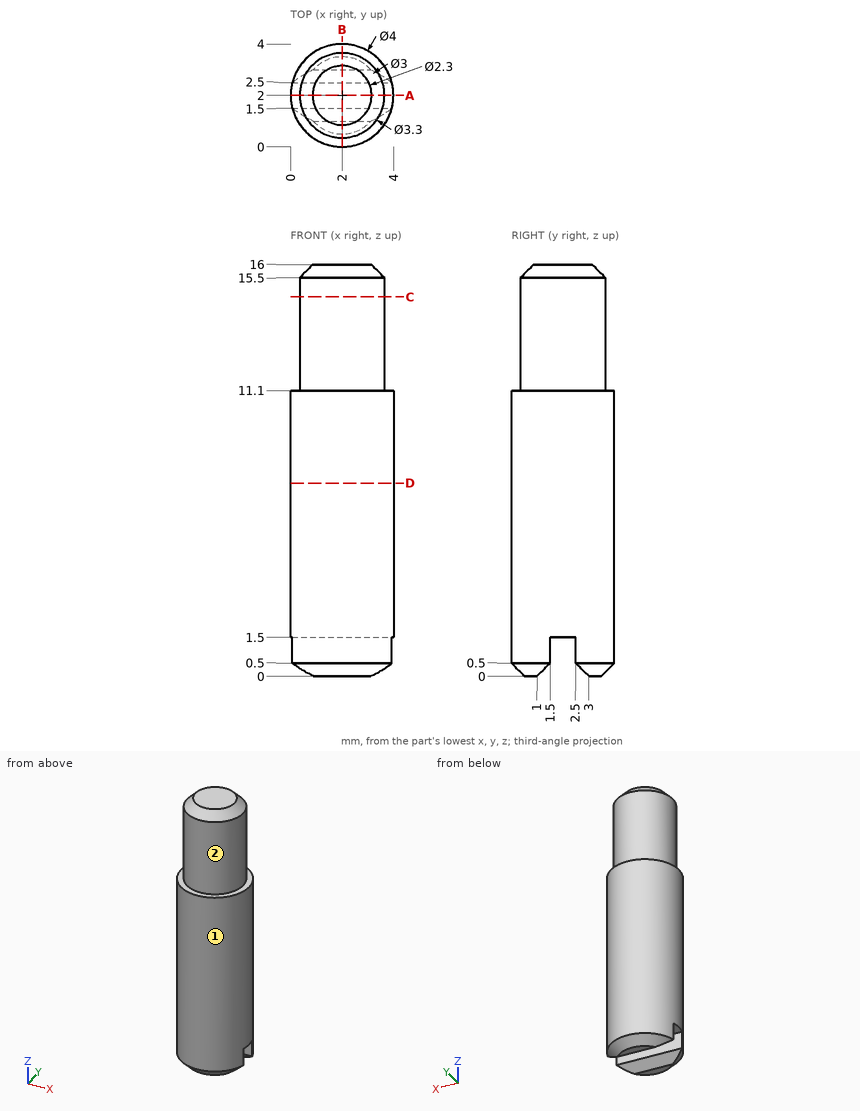
Geometry: see drawing. Coordinates: mm, zero at the bounding-box minimum. A direction names the side the tool comes from. Coordinates: 2 decimals unless noted, no trailing zeros. Loops run counter-clockwise (first coordinate to the right, second up) from the corner with the lowest first, then second, coordinate; pieces in that order, holes last. Notation, with made-up numbers: M -11.75,69 L 41.25,69 A21 ccw 41.25,78 Z; hole C 74,-29.5 d11. An arc over 180 degrees is marked long. Put each result on its own line as item: value. Start each with the question number.
1) Ray query, L1, parallel to Z at x = 1.4, y = 2.25; L2, parallel to Y at x = 2.8, z = 10; L3, parallel to X at y = 2.8, z = 13.5. Return the intervals inside material, ascending. Write a range as from..to.
2) Cut plane B-B on x = 2. Return the cut outline in (y, z).
3) Contact query for flat-ended pins moving along their axis: pin 1 Ø0.8 at (x, y) = (3, 2) entering from -Z; pin 2 Ø1.5 at (x, z) = (3, 14) entering from +Y. Output: stop coordinate, or through.
4) Cut plane A-A on y = 2. Return the cut outline in (x, z), then the cut area to 3 significant figures.
5) Reachability of the marked faces 1 and 2 from +Z, -Z, +X, -X, +Y, -Y: full face, straight path, thin tool, end or side. Return the list, or none.
6) Cut plane C-C on z = 14.75. Return the cut outline in (x, y), then the cut area to 3 significant figures.
7) Cut plane D-D on z = 7.5. Return the cut outline in (x, y), then the cut area to 3 significant figures.
The answers:
1. L1: z = 1.5..16
1. L2: y = 0.17..3.83
1. L3: x = 0.56..3.44
2. outline: M 0,0.5 L 0.5,0 L 1,0 L 1.5,0.5 L 1.5,1.5 L 2.5,1.5 L 2.5,0.5 L 3,0 L 3.5,0 L 4,0.5 L 4,11.1 L 3.65,11.1 L 3.65,15.5 L 3.15,16 L 0.85,16 L 0.35,15.5 L 0.35,11.1 L 0,11.1 Z
3. pin 1: stops at z = 1.5
3. pin 2: stops at y = 3.63
4. outline: M 0,1.5 L 4,1.5 L 4,11.1 L 3.65,11.1 L 3.65,15.5 L 3.15,16 L 0.85,16 L 0.35,15.5 L 0.35,11.1 L 0,11.1 Z
4. area: 54.3 mm²
5. face 1: +Z, -Z
5. face 2: +Z
6. outline: C 2,2 d3.3
6. area: 8.55 mm²
7. outline: C 2,2 d4
7. area: 12.6 mm²
